Geometry check sheet. Reference: the model listing, model coordinates, mm. A direction names the side the tool comes from. Round coordinates to 2 decimals unless told otherwise and drop trailing zeros. Write each loop counter-clockwise with the first axis right and the second up, starting at its lowest first coordinate (ties: lowest second). Pieces come first, ordered by that corner, then holes. Notation, with made-up numbers: (73.5, -34) - (114.5, -34) arc R25 ccw to (114.5, -18) - close; hole circle Ø2 at (77.25, 8). An arc over 180 degrees is marked (long way). Return JSON: item names as keys, results as strings. Group by question number.
from build123d import *

# Parameters (mm, degrees)
SKETCH_W        = 153
SKETCH_H        = 153
PAD_DEPTH       = 3
SKETCH001_W     = 153
SKETCH001_H     = 153
SKETCH001_W_2   = 147
SKETCH001_H_2   = 147
PAD001_DEPTH    = 122
SKETCH002_W     = 147
SKETCH002_H     = 20
POCKET_DEPTH    = 200
SKETCH003_W     = 137
SKETCH003_H     = 137
POCKET001_DEPTH = 5
SKETCH004_R     = 6.5
POCKET002_DEPTH = 3
SKETCH005_W     = 110
SKETCH005_H     = 20
POCKET003_DEPTH = 3


with BuildPart() as part:
    # Sketch → Pad (new body)
    with BuildSketch(Plane.XY):
        with Locations((76.5, 76.5)):
            Rectangle(SKETCH_W, SKETCH_H)
    extrude(amount=PAD_DEPTH)

    # Sketch001 (on Face6 of Pad) → Pad001 (join)
    with BuildSketch(Plane.XY.offset(3)):
        with Locations((76.5, 76.5)):
            Rectangle(SKETCH001_W, SKETCH001_H)
        with Locations((76.5, 76.5)):
            Rectangle(SKETCH001_W_2, SKETCH001_H_2, mode=Mode.SUBTRACT)
    extrude(amount=PAD001_DEPTH)

    # Sketch002 (on Face10 of Pad001) → Pocket (cut)
    with BuildSketch(Plane(origin=(0, 153, 0), x_dir=(-1, 0, 0), z_dir=(0, 1, 0))):
        with Locations((-76.5, 13)):
            Rectangle(SKETCH002_W, SKETCH002_H)
    extrude(amount=-POCKET_DEPTH, mode=Mode.SUBTRACT)

    # Sketch003 (on Face4 of Pocket) → Pocket001 (cut)
    with BuildSketch(Plane(origin=(0, 0, 0), x_dir=(1, 0, 0), z_dir=(0, 0, -1))):
        with Locations((76.5, -76.5)):
            Rectangle(SKETCH003_W, SKETCH003_H)
    extrude(amount=-POCKET001_DEPTH, mode=Mode.SUBTRACT)

    # Sketch004 (on Face8 of Pocket001) → Pocket002 (cut)
    with BuildSketch(Plane(origin=(0, 0, 0), x_dir=(0, -1, 0), z_dir=(-1, 0, 0))):
        with Locations((-75, 31)):
            Circle(SKETCH004_R)
    extrude(amount=-POCKET002_DEPTH, mode=Mode.SUBTRACT)

    # Sketch005 (on Face9 of Pocket002) → Pocket003 (cut)
    with BuildSketch(Plane.YZ.offset(153)):
        with Locations((76.5, 28)):
            Rectangle(SKETCH005_W, SKETCH005_H)
    extrude(amount=-POCKET003_DEPTH, mode=Mode.SUBTRACT)


solid = part.part
1. Material ranges on line 1 along X through (y, z) = (8, 30); line 2 along Z through (x, y) = (1, 75), recorded low to high.
2. Section check C-C (z = 31). Enter the section's corners in (x, y), and give its area (3 significant figures).
3. Section check D-D (y = 75). Enter the section's corners in (x, z).
4. Depth check by flat-ended pin: pin 1 Ø10.5 at (y, z) = (75, 31) entering from -X. Enter the tip coordinate at first touch or a pass-through.
5. Mould release check, pull along Y, two halves, no side actions. Record for faces 1 (the face through (1.48, 68.8, 32.95)), 2 (the face through (75, 0, 76)), 3 (the face through (148, 77, 3)), 4 (the face through (150, 75, 77)): pulls with the +Y half, pulls with the -Y half, needs draft (parallel to the pull), parting line crosses it, or undercut.
6. Tool access check on faces 5 (the face through (70, 3, 0)), 6 (the face through (75, 3, 73)). Record the directions out of +Z, -Z, +X, -X, +Y, -Y that give a thin tool (end or side, any length) a straight path to the whole face; none if there is none.
7. Section check B-B (x = 83). Enter the section's corners in (y, z), and give its area (3 significant figures).
8. Section check A-A (y = 114.5). Enter the section's corners in (x, z), and give its area (3 significant figures).
Result sheet:
{
 "1": {"line 1": "x = 0 to 3, 150 to 153", "line 2": "z = 0 to 24.5, 37.5 to 125"},
 "2": {"outline": "(0, 0) - (153, 0) - (153, 21.5) - (150, 21.5) - (150, 3) - (3, 3) - (3, 68.5) - (0, 68.5) - close; (0, 81.5) - (3, 81.5) - (3, 150) - (150, 150) - (150, 131.5) - (153, 131.5) - (153, 153) - (0, 153) - close", "area": "1,430 mm²"},
 "3": {"outline": "(0, 0) - (8, 0) - (8, 3) - (3, 3) - (3, 24.5) - (0, 24.5) - close; (0, 37.5) - (3, 37.5) - (3, 125) - (0, 125) - close; (145, 0) - (153, 0) - (153, 18) - (150, 18) - (150, 3) - (145, 3) - close; (150, 38) - (153, 38) - (153, 125) - (150, 125) - close"},
 "4": {"pin 1": "passes through"},
 "5": {"face 1": "undercut", "face 2": "pulls with the -Y half", "face 3": "needs draft", "face 4": "undercut"},
 "6": {"face 5": "-Z, +X, -X, +Y, -Y", "face 6": "+Z"},
 "7": {"outline": "(0, 0) - (8, 0) - (8, 3) - (0, 3) - close; (0, 23) - (3, 23) - (3, 125) - (0, 125) - close; (145, 0) - (153, 0) - (153, 3) - (145, 3) - close; (150, 23) - (153, 23) - (153, 125) - (150, 125) - close", "area": "660 mm²"},
 "8": {"outline": "(0, 0) - (8, 0) - (8, 3) - (3, 3) - (3, 125) - (0, 125) - close; (145, 0) - (153, 0) - (153, 18) - (150, 18) - (150, 3) - (145, 3) - close; (150, 38) - (153, 38) - (153, 125) - (150, 125) - close", "area": "720 mm²"}
}
